Design review of the part built by this model. Coordinates are the model's own, in mm. Face numbers are marked on the shaded views. Give positions to 0.01 mm unless a question says otherwise; leave off trailing zeros. Write each loop counter-clockwise with the first axis right and the second up, starting at its lowest first coordinate (ties: lowest second). Pieces come first, ordered by that corner, then holes. Notation, with made-up numbers: (89, -4.75) - (143, -4.75) arc R28 cw to (143, 27.25) - close; hole circle Ø9 at (7.25, -39.75). An arc over 180 degrees is marked (long way). Write each question's results on one line, items separated by ' | '. Start each with the question number.
from build123d import *

# Parameters (mm, degrees)
F2_DEPTH = 30
F4_DEPTH = 100
F6_R     = 15
F7_DEPTH = 50
F9_DEPTH = 100


with BuildPart() as f2:
    # F1 (on offset) → F2 (new body)
    with BuildSketch(Plane.XZ.offset(50)):
        with BuildLine():
            Line((100, 15), (-100, 15))
            ThreePointArc((-100, 15), (-115, 0), (-100, -15))
            Line((-100, -15), (100, -15))
            ThreePointArc((100, -15), (115, 0), (100, 15))
        make_face()
    extrude(amount=F2_DEPTH)

    # F3 (on face) → F4 (join)
    with BuildSketch(Plane.XZ.offset(80)):
        with BuildLine():
            ThreePointArc((0, -15), (10.606602, -10.606602), (15, 0))
            ThreePointArc((15, 0), (10.606602, 10.606602), (0, 15))
            ThreePointArc((0, 15), (-15, 0), (0, -15))
        make_face()
    extrude(amount=F4_DEPTH)

    # F6 (on face) → F7 (join)
    with BuildSketch(Plane(origin=(0, -50, 0), x_dir=(-1, 0, 0), z_dir=(0, 1, 0))):
        with Locations((-100, 0)):
            Circle(F6_R)
        with Locations((100, 0)):
            Circle(F6_R)
    extrude(amount=F7_DEPTH)

    # F8 (on Top) → F9 (join)
    with BuildSketch(Plane.XY):
        Polygon((-15, -180), (0, -180), (15, -180), (15, -150), (-15, -150), align=None)
    extrude(amount=-F9_DEPTH)


solid = f2.part
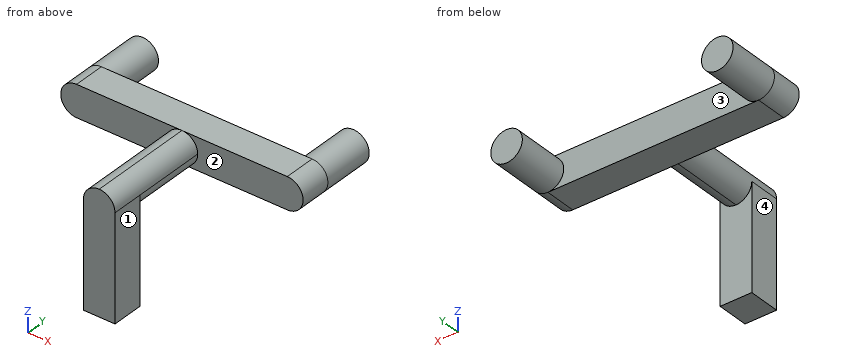
Q1. Add section C-C on y = -154.5. State the section outline as (x, z) points.
Q2. Add section D-D on x = 79.5. State the section outline as (y, z) points, plus the area to 3 significant figures.
Q3. The part is to be moulded in two halves that separate along X. For the marked faces 1, 2, 3 and 4, say which applies: +X half, -X half, draft (parallel to the pull), parting line (faces both ways), or undercut.
Q4. Insertion check: P1, Ø24, axis at x = 46, y = -63.5, coming from the -Z side; P2, Ø24, axis at x = 54.5, z = 6, coming from the -Y side; P3, Ø24, axis at x = 5, z = -45, coming from the +Y side. Each pin has a flat end and moves straight along its axis. Give the tip position at first contact, or say it passes through.
Q5. For line 1 along X through (y, z) = (-161.5, 0); line 2 along Y through (x, z) = (89, -12.5), list the stretches that pass through material, from the lowest coordinate up. Write a range as [from, to].
Q6. Add section A-A on y = -37.5. State the section outline as (x, z) points, plus the area to 3 significant figures.
Q7. Add section B-B on z = -10. State the section outline as (x, y) points, plus the area to 3 significant figures.
Result:
1) outline: (-15, -100) - (15, -100) - (15, 0) arc R15 ccw to (-15, 0) - close
2) outline: (-80, -15) - (-50, -15) - (-50, 15) - (-80, 15) - close | area: 900 mm²
3) face 1: +X half | face 2: draft | face 3: undercut | face 4: -X half
4) P1: stops at z = -15 | P2: stops at y = -80 | P3: stops at y = -150
5) line 1: x = [-15, 15] | line 2: y = [-80, -50]
6) outline: circle Ø30 at (-100, 0); circle Ø30 at (100, 0) | area: 1,410 mm²
7) outline: (-111.18, -80) - (-11.18, -80) - (-11.18, -150) - (-15, -150) - (-15, -180) - (15, -180) - (15, -150) - (11.18, -150) - (11.18, -80) - (111.18, -80) - (111.18, 0) - (88.82, 0) - (88.82, -50) - (-88.82, -50) - (-88.82, 0) - (-111.18, 0) - close | area: 11,400 mm²
